Can you work these out from the drawing? Everything is in mm from the part's minimum corner. Coordinates: 2 decimals unless noted, no trailing zeros. Write each loop counter-clockwise with the first axis right and the second up, starting at its lowest first coordinate (ties: lowest second). Pieces come first, ordered by that corner, then holes. Notation, with made-up numbers: (23, 61.25) - (77, 61.25) arc R19 ccw to (77, 93.25) - close; hole circle Ø2 at (-8.5, 64). An arc over 180 degrees is marked (long way). One line per question, with ' | ' between items. Start each with the question number.
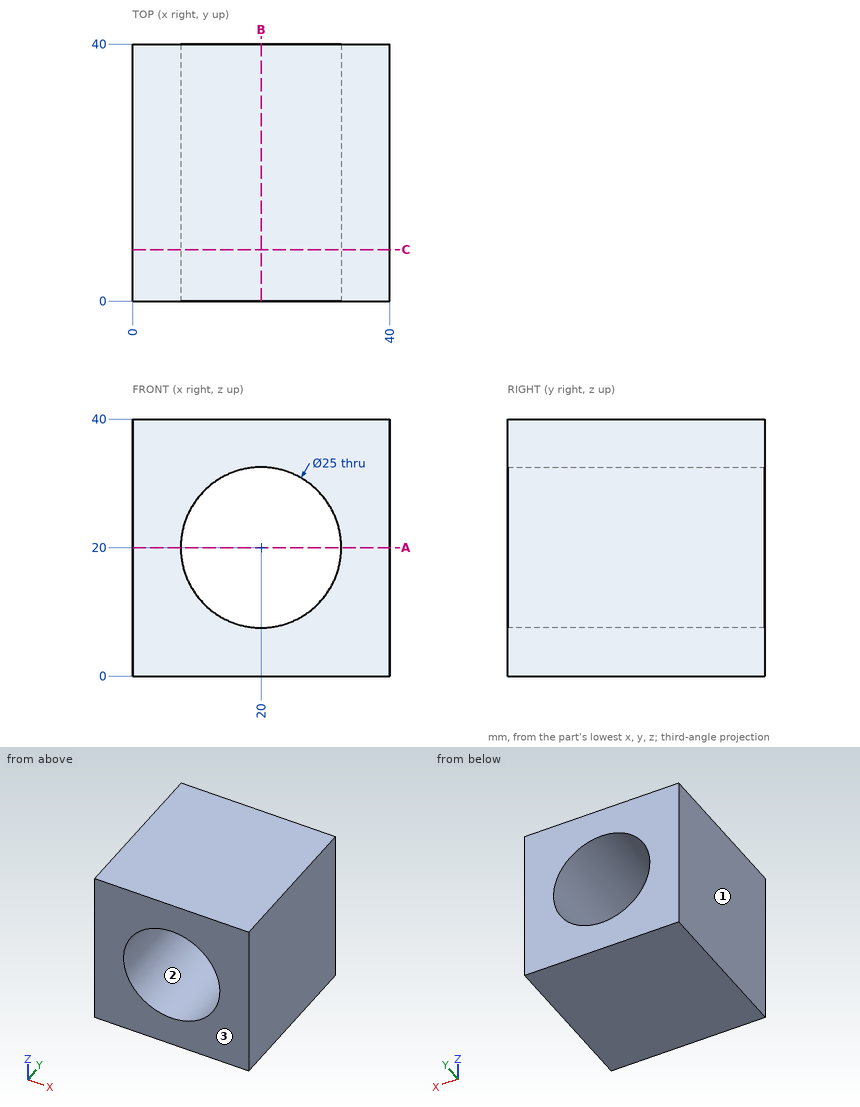
(1) If I drill on probe 1 along X at (y, z) = (19, 20); probe 2 along X at (y, z) = (9.5, 26.5), over which ranges is the centre line in solid material (lowest first)?
(2) If we section it at A-A on z = 20: List the corners of the cut face in (x, y) for me.
(3) If we mould it in two halves opening along X, with no side actions, what happens to the marked faces 1, 2 and 3? For each: +X half, -X half, draft (parallel to the pull), parting line (faces both ways), or undercut.
(4) If we section it at C-C on y = 8: List the corners of the cut face in (x, z) for me, plus the area to 3 significant figures.
(5) I'm going to push a flat-ended pin straight in: pin 1 (10 mm diameter, centred on x = 18.5, z = 23.5, fed in from +Y). Where does the tip first touch, or does it pass through?
(6) If we section it at B-B on x = 20: List the corners of the cut face in (y, z) for me, plus the area to 3 significant figures.
Values:
1) probe 1: 0 to 7.5, 32.5 to 40 | probe 2: 0 to 9.32, 30.68 to 40
2) outline: (0, 0) - (7.5, 0) - (7.5, 40) - (0, 40) - close; (32.5, 0) - (40, 0) - (40, 40) - (32.5, 40) - close
3) face 1: -X half | face 2: undercut | face 3: draft
4) outline: (0, 0) - (40, 0) - (40, 40) - (0, 40) - close; hole circle Ø25 at (20, 20) | area: 1,110 mm2
5) pin 1: through
6) outline: (0, 0) - (40, 0) - (40, 7.5) - (0, 7.5) - close; (0, 32.5) - (40, 32.5) - (40, 40) - (0, 40) - close | area: 600 mm2
